Autodesk Inventor part; units mm, degrees
ref_plane "YZ Plane" through (0, 0, 0) normal (1, 0, 0) x (0, 1, 0)
ref_plane "XZ Plane" through (0, 0, 0) normal (0, 1, 0) x (-1, 0, 0)
ref_plane "XY Plane" through (0, 0, 0) normal (0, 0, 1) x (1, 0, 0)
sketch "Sketch1" plane through (0, 0, 0) normal (0, 0, 1) x (1, 0, 0)
  line L0 (0, 0) -> (-30, 0)
  line L1 (-30, 0) -> (-30, 360)
  line L2 (-30, 360) -> (0, 360)
  line L3 (0, 360) -> (0, 0)
  line L4 (-40, 240) -> (10, 240)
  line L5 (10, 240) -> (10, 0)
  line L6 (10, 0) -> (-40, 0)
  line L7 (-40, 0) -> (-40, 240)
  line L8 (-50, 120) -> (20, 120)
  line L9 (20, 120) -> (20, 0)
  line L10 (20, 0) -> (-50, 0)
  line L11 (-50, 0) -> (-50, 120)
  line L12 (-5, 10) -> (-25, 10)
  line L13 (-25, 10) -> (-25, 15)
  line L14 (-25, 15) -> (-5, 15)
  line L15 (-5, 15) -> (-5, 10)
  line L16 (-25, 350) -> (-5, 350)
  line L17 (-5, 350) -> (-5, 345)
  line L18 (-5, 345) -> (-25, 345)
  line L19 (-25, 345) -> (-25, 350)
  dimension "d0" = 30
  dimension "d1" = 360
  dimension "d2" = 50
  dimension "d3" = 70
  dimension "d4" = 20
  dimension "d5" = 5
  dimension "d6" = 5
extrude "Extrusion1" add sketch "Sketch1" along normal blind 15
fillet "Fillet1" radius 5 4 edges at (-50, 0, 7.5) (20, 0, 7.5) (-30, 360, 7.5) (0, 360, 7.5)
properties part number "TENSOR"
The model under review builds one solid part; all positions refer to its coordinate system, in mm. A direction names the side the tool comes from. Give positions to 0.01 mm unless a question says otherwise; leave off trailing zeros. Write each loop counter-clockwise with the first axis right and the second up, starting at its lowest first coordinate (ties: lowest second). Pieces come first, ordered by that corner, then holes.
1. Add section B-B, the plane x = -18. Write out the cut boundary in (y, z), plus the area to 3 significant figures.
2. For P1, Ø4, axis at y = 347.5, z = 7.5, coming from the -X side; P2, Ø4.5, axis at y = 206.5, z = 10.5, coming from the +X side; P3, Ø5, axis at x = 15, z = 8, coming from the +Y side, all flat-tipped, find the tip position at first contact; note any pin that passes through.
3. Tool access review of faces 1 (the flat face through (-15, 15, 7)), 2 (the flat face through (-45, 120, 7)), 3 (the flat face through (0, 298, 7)): name each direction out of +Z, -Z, +X, -X, +Y, -Y from which nothing blocks a thin tool from reaching the whole face with its end or side.
4. Add section A-A, the plane z = 3. Write out the cut boundary in (x, y).
5. Draft analysis for pull direction X (two halves, no side actions). For faces 4 (the flat face through (-15, 350, 7)), 5 (the flat face through (-50, 62, 7)), 6 (the flat face through (-15, 345, 7)), 7 (the flat face through (20, 63, 7)), state which applies: +X half, -X half, draft (parallel to the pull), parting line (faces both ways), or undercut.
6. Wall thickness on L1, parallel to Y at x = -17, z = 5; L2, parallel to Y at x = -36.5, z = 2.25; L3, parallel to Y at x = -43, z = 2.25: over which ranges is each line inside the solid? List them lowest first.
7. Add section C-C, the plane y = 306. Write out the cut boundary in (x, z).
8. Add section D-D, the plane x = -37. Write out the cut boundary in (y, z).
Worked answers:
1. outline: (0, 0) - (10, 0) - (10, 15) - (0, 15) - close; (15, 0) - (345, 0) - (345, 15) - (15, 15) - close; (350, 0) - (360, 0) - (360, 15) - (350, 15) - close
1. area: 5,250 mm2
2. P1: stops at x = -30
2. P2: stops at x = 10
2. P3: stops at y = 120
3. face 1: +Z, -Z
3. face 2: +Z, -Z, -X, +Y
3. face 3: +Z, -Z, +X, +Y
4. outline: (-50, 5) arc R5 ccw to (-45, 0) - (15, 0) arc R5 ccw to (20, 5) - (20, 120) - (10, 120) - (10, 240) - (0, 240) - (0, 355) arc R5 ccw to (-5, 360) - (-25, 360) arc R5 ccw to (-30, 355) - (-30, 240) - (-40, 240) - (-40, 120) - (-50, 120) - close; hole (-25, 10) - (-5, 10) - (-5, 15) - (-25, 15) - close; hole (-25, 345) - (-5, 345) - (-5, 350) - (-25, 350) - close
5. face 4: undercut
5. face 5: -X half
5. face 6: undercut
5. face 7: +X half
6. L1: y = 0 to 10, 15 to 345, 350 to 360
6. L2: y = 0 to 240
6. L3: y = 0 to 120
7. outline: (-30, 0) - (0, 0) - (0, 15) - (-30, 15) - close
8. outline: (0, 0) - (240, 0) - (240, 15) - (0, 15) - close
